from build123d import *

# Parameters (mm, degrees)
F0_W      = 50.8
F0_H      = 44.45
F1_DEPTH  = 2254.25
F2_W      = 15.875
F2_H      = 22.225
F3_DEPTH  = 2260.6
F5_DEPTH  = 76.2
F11_DEPTH = 7.62
F13_DEPTH = 7.62
F15_DEPTH = 7.62
F17_DEPTH = 7.62


with BuildPart() as f1:
    # F0 (on Top) → F1 (new body)
    with BuildSketch(Plane.XY):
        with Locations((25.4, 22.225)):
            Rectangle(F0_W, F0_H)
    extrude(amount=F1_DEPTH)

    # F2 (on face) → F3 (cut)
    with BuildSketch(Plane.XY.offset(2254.25)):
        with Locations((17.4625, 33.3375)):
            Rectangle(F2_W, F2_H)
    extrude(amount=-F3_DEPTH, mode=Mode.SUBTRACT)

    # F4 (on face) → F5 (cut)
    with BuildSketch(Plane.YZ.offset(50.8)):
        Polygon((44.45, 3.8888710937), (0, 0), (44.45, 0), align=None)
    extrude(amount=-F5_DEPTH, mode=Mode.SUBTRACT)

    # F10 (on offset) → F11 (cut)
    with BuildSketch(Plane(origin=(0, -45.9354342152, 525.0444156293), x_dir=(1, 0, 0), z_dir=(0, 0.0871557427, -0.9961946981))):
        Polygon((68.3375078249, -83.8695270738), (52.6410068005, -68.1730260494), (29.9672586024, -90.8467742476), (45.6637596268, -106.543275272), align=None)
    extrude(amount=-F11_DEPTH, mode=Mode.SUBTRACT)

    # F12 (on offset) → F13 (cut)
    with BuildSketch(Plane(origin=(0, -65.0290785576, 743.2857691137), x_dir=(1, 0, 0), z_dir=(0, 0.0871557427, -0.9961946981))):
        Polygon((50.8, -93.1639036529), (30.0833409598, -111.4171829045), (48.0814183777, -131.8441992288), (68.7980774179, -113.5909199772), align=None)
    extrude(amount=-F13_DEPTH, mode=Mode.SUBTRACT)

    # F14 (on offset) → F15 (cut)
    with BuildSketch(Plane(origin=(0, -102.662928276, 1173.4426397497), x_dir=(1, 0, 0), z_dir=(0, 0.0871557427, -0.9961946981))):
        Polygon((50.8, -128.6248757626), (31.75, -147.6748757626), (46.4404728378, -162.3653486004), (65.4904728378, -143.3153486004), align=None)
    extrude(amount=-F15_DEPTH, mode=Mode.SUBTRACT)

    # F16 (on offset) → F17 (cut)
    with BuildSketch(Plane(origin=(0, -144.7242897261, 1654.2062010488), x_dir=(1, 0, 0), z_dir=(0, 0.0871557427, -0.9961946981))):
        Polygon((50.8, -170.8469047802), (31.75, -189.8969047802), (46.5661471594, -204.7130519396), (65.6161471594, -185.6630519396), align=None)
    extrude(amount=F17_DEPTH, mode=Mode.SUBTRACT)


solid = f1.part
Model file for the job. Use its own axes, mm. Give positions to 0.01 mm unless a question says otherwise; leave off trailing zeros. Loops run counter-clockwise (first coordinate to the right, second up) from the corner with the lowest first, then second, coordinate; pieces in that order, holes last. Notation, with made-up numbers: (56, -29) -> (79, -29) arc R17 ccw to (79, 4) -> close; hole circle Ø2 at (79.25, 46.5). An arc over 180 degrees is marked (long way). Use a Markdown table: item, result. Add a question column.
(1) Slice it at B-B on z = 1333. List the corners of the cut face in (x, y) (3 decimals).
(2) Drop flat-ended pins along their axis: pin 1 Ø5 at (x, z) = (22, 1295) entering from +Y (3 decimals); pin 2 Ø6 at (x, y) = (44.5, 19.5) entering from -Z. Give the stop position or say it passes through.
(3) Slice it at A-A on y = 36.5. List the corners of the cut face in (x, z) (3 decimals).
(4) Wall check: line 1 along X through (y, z) = (30.5, 114) (3 decimals); line 2 along Y through (x, z) = (18.5, 2045.5) (3 decimals); line 3 along Z through (x, y) = (12, 4.5). Give the ranges that are in metal, low to high.
Filled sheet:
| question | item | result |
|---|---|---|
| 1 | outline | (0, 0) -> (50.8, 0) -> (50.8, 44.45) -> (25.4, 44.45) -> (25.4, 22.225) -> (9.525, 22.225) -> (9.525, 44.45) -> (0, 44.45) -> close |
| 2 | pin 1 | y = 22.225 |
| 2 | pin 2 | z = 1.44 |
| 3 | outline | (0, 3.193) -> (9.525, 3.193) -> (9.525, 2254.25) -> (0, 2254.25) -> close; (25.4, 3.193) -> (50.8, 3.193) -> (50.8, 532.257) -> (38.064, 532.257) -> (37.397, 539.906) -> (50.8, 539.906) -> (50.8, 752.168) -> (40.866, 752.168) -> (40.109, 759.818) -> (50.8, 759.818) -> (50.8, 1185.618) -> (39.73, 1185.618) -> (39.064, 1193.267) -> (50.8, 1193.267) -> (50.8, 1662.412) -> (40.397, 1662.412) -> (39.73, 1670.061) -> (50.8, 1670.061) -> (50.8, 2254.25) -> (25.4, 2254.25) -> close |
| 4 | line 1 | 0 to 9.525, 25.4 to 50.8 |
| 4 | line 2 | 0 to 22.225 |
| 4 | line 3 | 0.39 to 2254.25 |
